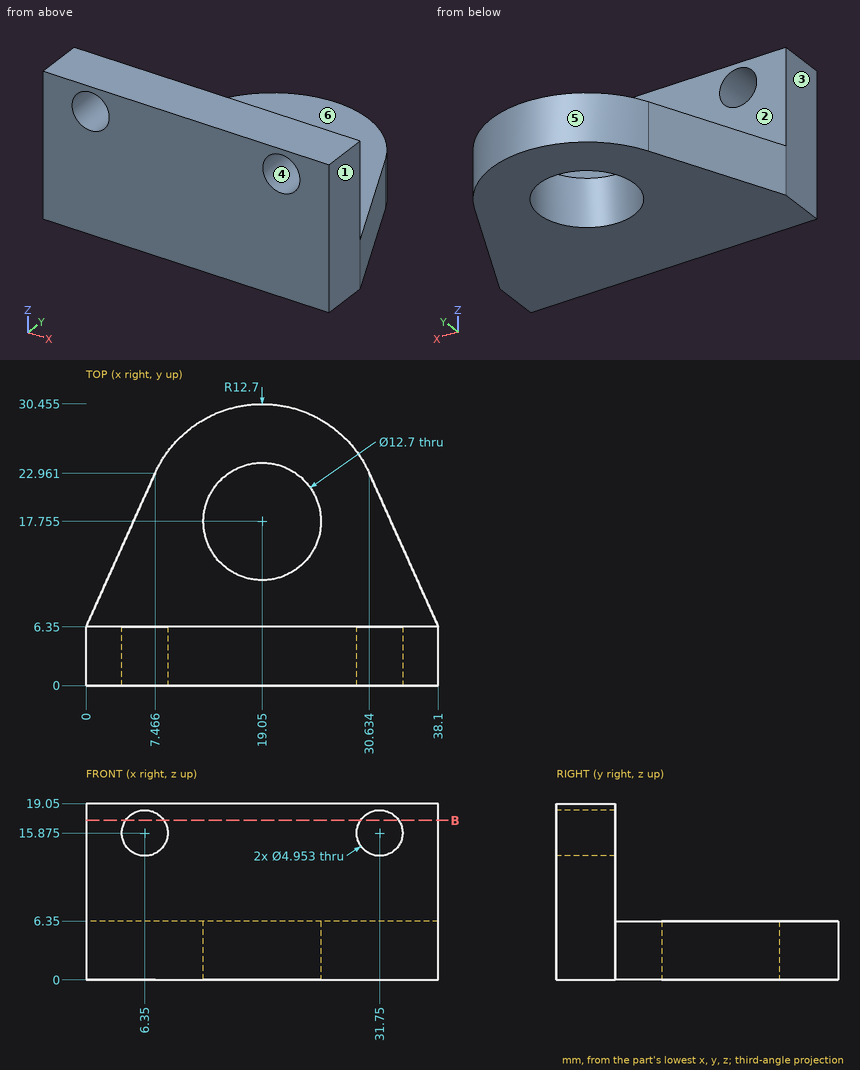
Could you check a few things on this drawing? It's one solid part, dimensions in mm from its lowest x, y, z. A direction names the side the tool comes from. Coordinates: 2 decimals unless noted, no trailing zeros. Write each loop counter-clockwise with the first axis right and the second up, starting at its lowest first coordinate (ties: lowest second). Pieces come first, ordered by that corner, then holes.
1) Which directions (+Z, -Z, +X, -X, +Y, -Y) give clear straight access to the entire face, cutting with the end or side of a thin tool? Please do the marked faces 5 and 6.
Filled in:
face 5: +Z, -Z, +Y
face 6: +Z, +X, -X, +Y
2) Thinking about a two-plate mould opening in X: for the marked faces 1, 2, 3 and 4, which applies, +X half, -X half, draft (parallel to the pull), parting line (faces both ways), or undercut?
Filled in:
face 1: +X half
face 2: draft
face 3: -X half
face 4: undercut
3) If I drill on line 1 (Z direction, x = 31.75, y = 3.75); line 2 (Y direction, x = 19.05, z = 4.25) (1 decimal); line 3 (Y direction, x = 23.5, z = 13), over which ranges is the centre line in solid material (lowest first)?
Filled in:
line 1: z = 0 to 13.4, 18.35 to 19.05
line 2: y = 0 to 11.4, 24.1 to 30.5
line 3: y = 0 to 6.35
4) I'm going to push flat-ended pins straight in: pin 1 (5.5 mm diameter, centred on x = 6.35, z = 15.875, fed in from +Y); pin 2 (7 mm diameter, centred on x = 23, y = 21, fed in from +Z); pin 3 (8 mm diameter, centred on y = 17.5, z = 7, fed in from +X). Where does each tip first touch, or does it pass through?
Filled in:
pin 1: stops at y = 6.35
pin 2: stops at z = 6.35
pin 3: stops at x = 34.86
5) If we section it at B-B (z = 17.25): List the corners of the cut face in (x, y) for me.
Filled in:
outline: (0, 0) - (4.29, 0) - (4.29, 6.35) - (0, 6.35) - close; (8.41, 0) - (29.69, 0) - (29.69, 6.35) - (8.41, 6.35) - close; (33.81, 0) - (38.1, 0) - (38.1, 6.35) - (33.81, 6.35) - close
